Autodesk Inventor part; units mm, degrees
ref_plane "YZ Plane" through (0, 0, 0) normal (1, 0, 0) x (0, 1, 0)
ref_plane "XZ Plane" through (0, 0, 0) normal (0, 1, 0) x (-1, 0, 0)
ref_plane "XY Plane" through (0, 0, 0) normal (0, 0, 1) x (1, 0, 0)
sketch "Esquisse1" plane through (0, 0, 0) normal (0, 0, 1) x (1, 0, 0)
  line L0 (0, -14) -> (0, 14) construction
  circle A0 centre (0, 0) radius 30 construction
  line L1 (0, 0) -> (35, 0) construction
  line L2 (0, 0) -> (-35, 0) construction
  line L3 (-35, 0) -> (35, 0) construction
  line L4 (35, 0) -> (35, -50)
  line L5 (-35, -50) -> (-35, 0)
  line L6 (-49, 0) -> (49, 0) construction
  line L7 (0, -66) -> (0, 46) construction
  arc A1 (-21.6, 0) -> (21.6, 0) centre (0, 0) ccw
  line L8 (-35, 0) -> (-21.6, 0)
  line L9 (35, 0) -> (21.6, 0)
  line L10 (-17, -50) -> (-17, -45)
  line L11 (-17, -45) -> (-27, -45)
  line L12 (-27, -45) -> (-27, -50)
  line L13 (27, -50) -> (27, -45)
  line L14 (27, -45) -> (17, -45)
  line L15 (17, -45) -> (17, -50)
  line L16 (-27, -50) -> (-35, -50)
  line L17 (35, -50) -> (27, -50)
  line L18 (17, -50) -> (-17, -50)
  line L19 (0, 0) -> (21.6, 0) construction
  line L20 (30, 0) -> (35, 0) construction
  dimension "d8" = 60
  dimension "d12" = 70
  dimension "d23" = 35
  dimension "d25" = 21.6
  dimension "d26" = 10
  dimension "d28" = 10
  dimension "d30" = 8
  dimension "d31" = 8
  dimension "d32" = 5
  dimension "d33" = 5
  dimension "d34" = 5
  dimension "d35" = 50
  dimension "d36" = 5
extrude "Extrusion1" add sketch "Esquisse1" along normal blind 3
properties part number "Support_motor_front_2"
Verification items for the finished model (mm, model axes). A direction names the side the tool comes from. Give positions to 0.01 mm unless a question says otherwise; leave off trailing zeros. Write each loop counter-clockwise with the first axis right and the second up, starting at its lowest first coordinate (ties: lowest second). Pieces come first, ordered by that corner, then holes. Notation, with made-up numbers: M -5,30.25 L 42,30.25 A12 ccw 42,49.25 Z; hole C 7,76 d2. An arc over 180 degrees is marked long. Write item = value, one per line.
(1) Draft check along X on faces 3 (the face through (35, -25, 1)), 4 (the face through (-31, -50, 1)), 5 (the face through (22, -45, 1)). Enter one of: released by +X, released by -X, zero draft, split by the parting line, or undercut.
Found:
face_3 = released by +X
face_4 = zero draft
face_5 = undercut
(2) Sectioned sample at A-A (y = -6.5). Record the cut outline in (x, z).
Found:
outline = M -35,0 L -20.6,0 L -20.6,3 L -35,3 Z; M 20.6,0 L 35,0 L 35,3 L 20.6,3 Z
(3) Sectioned sample at D-D (x = 20.5). Record the cut outline in (y, z).
Found:
outline = M -45,0 L -6.81,0 L -6.81,3 L -45,3 Z
(4) Sectioned sample at C-C (x = 0). Record the cut outline in (y, z), then the cut area to 3 significant figures.
Found:
outline = M -50,0 L -21.6,0 L -21.6,3 L -50,3 Z
area = 85.2 mm2
(5) Material ranges on line 1 (Y direction, x = -24.5, z = 2.5); line 2 (X direction, y = -14.5, z = 0.35); line 3 (X direction, y = -5, z = 2.75), recorded low to high.
Found:
line_1 = -45 to 0
line_2 = -35 to -16.01, 16.01 to 35
line_3 = -35 to -21.01, 21.01 to 35
(6) Sectioned sample at B-B (z = 2.45). Record the cut outline in (x, y).
Found:
outline = M -35,-50 L -27,-50 L -27,-45 L -17,-45 L -17,-50 L 17,-50 L 17,-45 L 27,-45 L 27,-50 L 35,-50 L 35,0 L 21.6,0 A21.6 cw -21.6,0 L -35,0 Z
(7) Access from +Z, -Z, +X, -X, +Y, -Y to the whole of each face (thin tool, end or side, straight path). Record for faces 1 (the face through (17, -47, 1)), 2 (the face through (0, -50, 1)).
Found:
face_1 = +Z, -Z, -Y
face_2 = +Z, -Z, +X, -X, -Y
